Geometry check sheet. Reference: the model listing, model coordinates, mm. A direction names the side the tool comes from. Give positions to 0.01 mm unless a question says otherwise; leave off trailing zeros. Loops run counter-clockwise (first coordinate to the right, second up) from the corner with the lowest first, then second, coordinate; pieces in that order, holes last. Notation, with made-up numbers: (41.5, 33) - (95.5, 33) arc R25 cw to (95.5, 55) - close; hole circle Ø5 at (-18, 10.25). An arc over 180 degrees is marked (long way). Use a Markdown table: item, result. Add a question column.
1. Draft check along Y on faces 1 (the flat face through (49.8, -0.8, 0.1)), 2 (the cylindrical face through (11.67, -0.07, -1.5)), 3 (the flat face through (46.8, 0, 0)), 4 (the flat face through (0.55, 1.5, 0.7)). Enter one of: pulls with the +Y half, pulls with the -Y half, needs draft (parallel to the pull), parting line crosses it, or undercut.
2. Cross-section at B-B on y = -2.5. Count the separate pieces of the cut face and the enclosed holes in it, and give its area (3 significant figures).
3. Depth check by flat-ended pin: P1, Ø3, axis at x = 47, y = 2, coming from the +Z side; P2, Ø3, axis at x = 30, z = 3, coming from the -Y side; P3, Ø3, axis at x = 31, z = -2.5, coming from the +Y side. Enter the tip coordinate at first touch or a pass-through.
4. Cross-section at D-D on x = 34.5. Enter the section's corners in (y, z).
5. Material ranges on L1, parallel to X at y = 0.5, z = -1.25; L2, parallel to X at y = 1.5, z = -1; L3, parallel to X at y = 2, z = 2.5, recorded low to high.
6. Cross-section at C-C on x = 21.5. Enter the section's corners in (y, z), and give its area (3 significant figures).
7. Cross-section at A-A on x = 51.45. Enter the section's corners in (y, z), and give its area (3 significant figures).
8. Set-up check for faces 5 (the cylindrical face through (44.84, -0.94, 2.98)), 6 (the flat face through (-0.008, 2.517, -1.136)), 7 (the flat face through (49.8, 0.8, -0.1)): record each of +Z, -Z, +X, -X, +Y, -Y from which the full face is reachable in a straight line by a thin tool's end or side.
from build123d import *

# Parameters (mm, degrees)
F3_DEPTH = 7.7
F4_R     = 1.35
F5_DEPTH = 12.5
F7_DEPTH = 0.55


with BuildPart() as f1:
    # F0 (on Front) → F1 (revolve)
    with BuildSketch(Plane.XZ):
        Polygon((0, 1.5), (0, 0), (54.5, 0), (54.5, 3.7), (45.3, 3.7), (45.3, 3.125), (44.4, 3.125), (44.4, 3.7), (27.8, 3.7), (27.8, 3.1), (23.1, 1.5), align=None)
    revolve(axis=Axis((27.25, 0, 0), (1, 0, 0)))

    # F2 (on face) → F3 (cut)
    with BuildSketch(Plane.YZ.offset(54.5)):
        with BuildLine():
            Line((0, -3.7), (0, 0))
            Line((0, 0), (0, 3.7))
            ThreePointArc((0, 3.7), (-0.4023866409, 3.6780545117), (-0.8, 3.6124783736))
            Line((-0.8, 3.6124783736), (-0.8, -3.6124783736))
            ThreePointArc((-0.8, -3.6124783736), (-0.4023866409, -3.6780545117), (0, -3.7))
        make_face()
        with BuildLine():
            Line((0, 3.7), (0, 0))
            Line((0, 0), (0, -3.7))
            ThreePointArc((0, -3.7), (0.4023866409, -3.6780545117), (0.8, -3.6124783736))
            Line((0.8, -3.6124783736), (0.8, 3.6124783736))
            ThreePointArc((0.8, 3.6124783736), (0.4023866409, 3.6780545117), (0, 3.7))
        make_face()
    extrude(amount=-F3_DEPTH, mode=Mode.SUBTRACT)

    # F4 (on Front) → F5 (cut, symmetric)
    with BuildSketch(Plane.XZ):
        with Locations((51.45, 0)):
            Circle(F4_R)
    extrude(amount=F5_DEPTH, both=True, mode=Mode.SUBTRACT)

    # F6 (on face) → F7 (join, symmetric)
    with BuildSketch(Plane(origin=(0, 0, 0), x_dir=(0, -1, 0), z_dir=(-1, 0, 0))):
        Polygon((3.1754264805, -0.2916945049), (1.8403280916, 2.6041527476), (-1.3350983889, 2.8958472524), (-3.1754264805, 0.2916945049), (-1.8403280916, -2.6041527476), (1.3350983889, -2.8958472524), align=None)
    extrude(amount=F7_DEPTH, both=True)


solid = f1.part
Values found:
| question | item | result |
|---|---|---|
| 1 | face 1 | undercut |
| 1 | face 2 | parting line crosses it |
| 1 | face 3 | undercut |
| 1 | face 4 | needs draft |
| 2 | separate pieces | 2 |
| 2 | enclosed holes | 1 |
| 2 | area | 145 mm2 |
| 3 | P1 | stops at z = 3.66 |
| 3 | P2 | stops at y = -3.38 |
| 3 | P3 | stops at y = 3.56 |
| 4 | outline | circle Ø7.4 at (0, 0) |
| 5 | L1 | x = -0.55 to 46.8 |
| 5 | L2 | x = -0.55 to 0.55, 23.99 to 50.54, 52.36 to 54.5 |
| 5 | L3 | x = 27.8 to 44.4, 45.3 to 54.5 |
| 6 | outline | circle Ø3 at (0, 0) |
| 6 | area | 7.07 mm2 |
| 7 | outline | (-3.44, -1.35) arc R3.7 ccw to (-0.8, -3.61) - (-0.8, -1.35) - close; (-3.44, 1.35) - (-0.8, 1.35) - (-0.8, 3.61) arc R3.7 ccw to start; (0.8, -3.61) arc R3.7 ccw to (3.44, -1.35) - (0.8, -1.35) - close; (0.8, 1.35) - (3.44, 1.35) arc R3.7 ccw to (0.8, 3.61) - close |
| 7 | area | 16.1 mm2 |
| 8 | face 5 | none |
| 8 | face 6 | -Z, -X, +Y |
| 8 | face 7 | +Z, -Z, +X |
